```python
from build123d import *

# Parameters (mm, degrees)
SKETCH_1_W               = 11
SKETCH_1_H               = 3.779
CUT_EXTRUDE_2_REACH      = 16.591
PATTERN_CIRCULAR_3_COUNT = 15
EXTRUDE_START            = 2
SKETCH_7_R               = 9
SKETCH_7_R_2             = 3
EXTRUDE_1_DEPTH          = 2
EXTRUDE_START_2          = -11
SKETCH_7_2_R             = 9
SKETCH_7_2_R_2           = 3
EXTRUDE_2_DEPTH          = 2
CHAMFER_1_SIZE           = 0.3


with BuildPart() as part:
    # 草图1 → 旋转1 (revolve)
    with BuildSketch(Plane.XY, mode=Mode.PRIVATE) as revolve_1_sk:
        with Locations((5.5, 4.8895)):
            Rectangle(SKETCH_1_W, SKETCH_1_H)
    revolve(revolve_1_sk.sketch.rotate(Axis((0, 0, 0), (1, 0, 0)), 90), axis=Axis((0, 0, 0), (1, 0, 0)))

    # 草图6 → 切除-拉伸2 (cut, up to next)
    with BuildSketch(Plane(origin=(0, 0, 0), x_dir=(0, 0, -1), z_dir=(1, 0, 0)), mode=Mode.PRIVATE) as cut_extrude_2_sk1:
        with BuildLine():
            Line((0.921029279, 6.443168288), (0.903216998, 6.298098898))
            ThreePointArc((0.903216998, 6.298098898), (0, 5.499), (-0.903216998, 6.298098898))
            Line((-0.903216998, 6.298098898), (-0.921029279, 6.443168288))
            ThreePointArc((-0.921029279, 6.443168288), (-1.025205225, 6.62105106), (-1.226117469, 6.667194084))
            ThreePointArc((-1.226117469, 6.667194084), (-1.353747907, 6.642454938), (-1.480880455, 6.615272789))
            Line((-1.480880455, 6.615272789), (-1.677528444, 8.216842132))
            ThreePointArc((-1.677528444, 8.216842132), (0, 8.386333901), (1.677528444, 8.216842132))
            Line((1.677528444, 8.216842132), (1.480880455, 6.615272789))
            ThreePointArc((1.480880455, 6.615272789), (1.353747907, 6.642454938), (1.226117469, 6.667194084))
            ThreePointArc((1.226117469, 6.667194084), (1.025205225, 6.62105106), (0.921029279, 6.443168288))
        make_face()
    cut_extrude_2_tool1 = extrude(cut_extrude_2_sk1.sketch, amount=CUT_EXTRUDE_2_REACH, mode=Mode.PRIVATE) & part.part
    cut_extrude_2 = cut_extrude_2_tool1.solids().sort_by_distance((0, 7.172733, 0))[0]
    add(cut_extrude_2, mode=Mode.SUBTRACT)

    # 阵列(圆周)3: 切除-拉伸2 ×15 about axis
    pattern_circular_3_axis = Axis((0, 0, 0), (1, 0, 0))
    for i in range(1, PATTERN_CIRCULAR_3_COUNT):
        add(cut_extrude_2.rotate(pattern_circular_3_axis, i * 360 / PATTERN_CIRCULAR_3_COUNT), mode=Mode.SUBTRACT)

    # 草图7 → 凸台-拉伸1 (add)
    with BuildSketch(Plane.ZY.offset(EXTRUDE_START)):
        Circle(SKETCH_7_R)
        Circle(SKETCH_7_R_2, mode=Mode.SUBTRACT)
    extrude(amount=-EXTRUDE_1_DEPTH)

    # 草图7<2> → 凸台-拉伸2 (add)
    with BuildSketch(Plane.ZY.offset(EXTRUDE_START_2)):
        Circle(SKETCH_7_2_R)
        Circle(SKETCH_7_2_R_2, mode=Mode.SUBTRACT)
    extrude(amount=-EXTRUDE_2_DEPTH)

    # 倒角1
    chamfer_1_edges = [part.edges().sort_by_distance(p)[0] for p in [
        (-2, 0, -9),
        (0, 0, -9),
        (-2, 0, -3),
        (13, 0, -9),
        (13, 0, -3),
        (11, 0, -9),
    ]]
    chamfer(chamfer_1_edges, length=CHAMFER_1_SIZE)


solid = part.part
```
The listing builds one solid part. Answer for the finished solid, in the listing's coordinates (mm). A direction names the side the tool comes from. Round coordinates to 2 decimals unless told otherwise and drop trailing zeros. Write each loop counter-clockwise with the first axis right and the second up, starting at its lowest first coordinate (ties: lowest second). Pieces come first, ordered by that corner, then holes. Notation, with made-up numbers: (85.25, 26.25) -> (103.25, 26.25) arc R18 ccw to (103.25, 57.25) -> close; hole circle Ø7 at (13, -26). An arc over 180 degrees is marked (long way). Answer as a JSON object with one key per item and string values. Group by question number.
Q1. Each of these flat-tipped pins is pushed along its axis until it touches: pin 1 Ø6 at (x, z) = (6, 3) entering from +Y; pin 2 Ø8 at (x, y) = (7.5, -5) entering from -Z; pin 3 Ø6 at (x, y) = (9.5, 3) entering from -Z. Where does it stop, or does it pass through?
Q2. Section A-A (y = 0) is taken. Write down the section's boundary in (x, z), plus the area to 3 significant figures.
Q3. Straight lines are drawn through the part: line 1 along X through (y, z) = (2.5, -5.5); line 2 along Y through (x, z) = (6.75, 0); line 3 along Y through (x, z) = (6.5, -0.75). For each, find the intervals that lie inside material, in ascending order.
Q4. Which of the six approach directions +Z, -Z, +X, -X, +Y, -Y give full straight-line access (tool end or side, diameter ignored) to faces 1 (the face through (5, 0, -3)), 2 (the face through (5.42, -4.46, -3.22))?
Q5. Determine the mould class of faces 3 (the face through (-1.01, 8.923, -1.172)), 4 (the face through (-2, 0, 4)), 5 (the face through (5.423, -0.593, -5.467)) for opening direction Y: pulls with the +Y half, pulls with the -Y half, needs draft (parallel to the pull), parting line crosses it, or undercut.
Check values:
{
 "1": {"pin 1": "y = 6.67", "pin 2": "z = -8.19", "pin 3": "z = -8.98"},
 "2": {"outline": "(-2, -8.7) -> (-1.7, -9) -> (-0.3, -9) -> (0, -8.7) -> (0, -5.76) -> (11, -5.76) -> (11, -8.7) -> (11.3, -9) -> (12.7, -9) -> (13, -8.7) -> (13, -3.3) -> (12.7, -3) -> (-1.7, -3) -> (-2, -3.3) -> close; (-2, 3.3) -> (-1.7, 3) -> (12.7, 3) -> (13, 3.3) -> (13, 8.7) -> (12.7, 9) -> (11.3, 9) -> (11, 8.7) -> (11, 5.76) -> (0, 5.76) -> (0, 8.7) -> (-0.3, 9) -> (-1.7, 9) -> (-2, 8.7) -> close", "area": "108 mm^2"},
 "3": {"line 1": "-2 to 0, 11 to 13", "line 2": "-6.78 to -3, 3 to 5.5", "line 3": "-5.57 to -2.9, 2.9 to 5.89"},
 "4": {"face 1": "+X, -X", "face 2": "none"},
 "5": {"face 3": "parting line crosses it", "face 4": "needs draft", "face 5": "undercut"}
}
